Input: dimensioned drawing with shaded views. Units: mm. Origin: part minimum x, y, z. Give positions to 0.01 mm unless a question says otherwise; leave off trailing zeros. Write each loop counter-clockwise with the first axis right and the second up, starting at its lowest first coordinate (ties: lowest second). Pieces come first, ordered by that corner, then holes.
Q1. Pin query (flat end, axial travel): pin 1 Ø1.5 at (y, z) = (2.5, 5) entering from +X; pin 2 Ø1 at (x, y) = (10, 0.5) entering from +Z; pin 3 Ø2 at (x, y) = (1.5, 2) entering from +Z. Return the tip coordinate at first contact, or that it passes through.
Q2. Mould query, pull axis X, two halves, no side actions, for the marked faces 1, 2, 3 and 4. Classes: +X half, -X half, draft (parallel to the pull), parting line (faces both ways), or undercut.
Q3. Section C-C (x = 5). Return the cut outline in (y, z), plus the area to 3 significant figures.
Q4. Section A-A (z = 6.5). Return the cut outline in (x, y), plus the area to 3 significant figures.
Q5. Section D-D (z = 1.5). Return the cut outline in (x, y), plus the area to 3 significant figures.
Q6. Section B-B (x = 6.5). Return the cut outline in (y, z), plus the area to 3 significant figures.
Q7. Line query: line 1 (X direction, y = 3.05, z = 6.5); line 2 (X direction, y = 0.85, z = 8.25); line 3 (Z direction, x = 1.25, y = 1.2). Output: solid intervals per line, ascending.
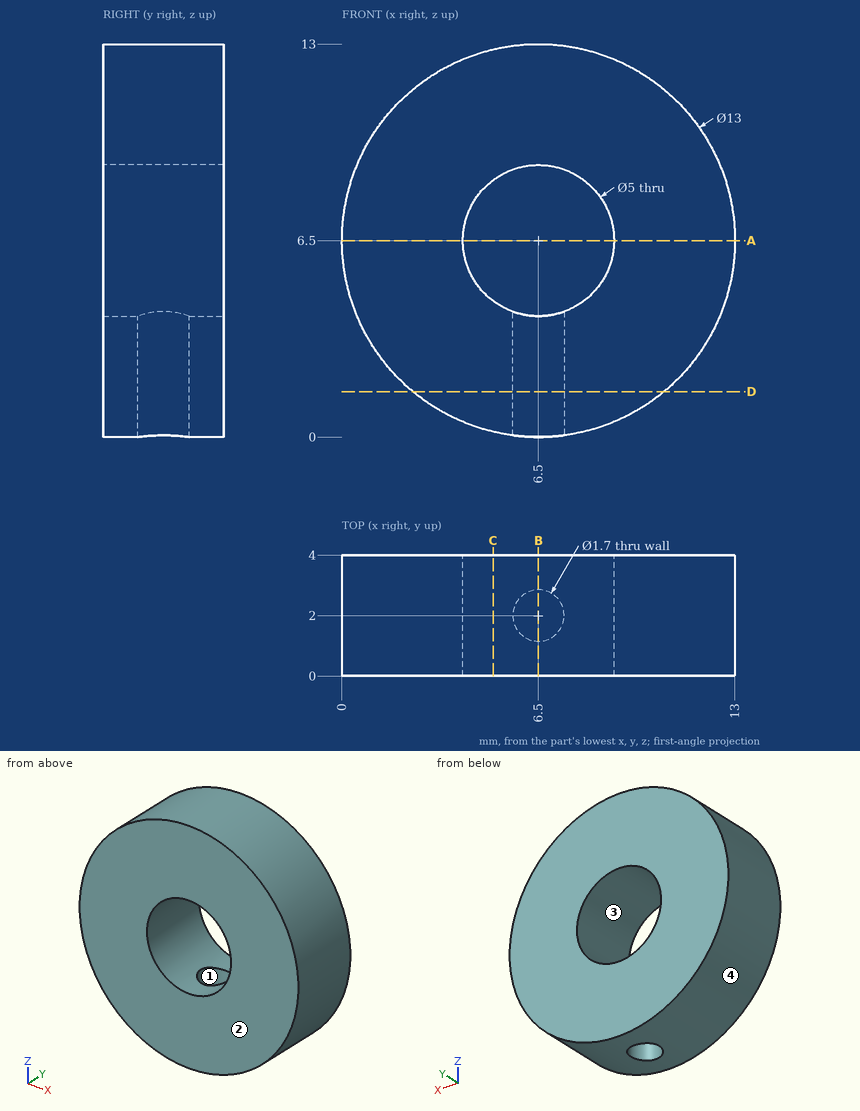
Computed:
1. pin 1: stops at x = 12.96
1. pin 2: stops at z = 12.27
1. pin 3: stops at z = 11.62
2. face 1: undercut
2. face 2: draft
2. face 3: undercut
2. face 4: parting line
3. outline: (0, 0.18) - (4, 0.18) - (4, 4.5) - (0, 4.5) - close; (0, 8.5) - (4, 8.5) - (4, 12.82) - (0, 12.82) - close
3. area: 34.6 mm2
4. outline: (0, 0) - (4, 0) - (4, 4) - (0, 4) - close; (9, 0) - (13, 0) - (13, 4) - (9, 4) - close
4. area: 32.0 mm2
5. outline: (2.35, 0) - (10.65, 0) - (10.65, 4) - (2.35, 4) - close; hole circle Ø1.7 at (6.5, 2)
5. area: 31.0 mm2
6. outline: (0, 0) - (1.15, 0) - (1.15, 4) - (0, 4) - close; (0, 9) - (4, 9) - (4, 13) - (0, 13) - close; (2.85, 0) - (4, 0) - (4, 4) - (2.85, 4) - close
6. area: 25.2 mm2
7. line 1: x = 0 to 4, 9 to 13
7. line 2: x = 0.24 to 4.71, 8.29 to 12.76
7. line 3: z = 2.67 to 10.33
